Part print with two shaded views. Sizes in mm from the minimum x, y, z corner. A direction names the side the tool comes from. Round coordinates to 2 decimals unless told otherwise and drop trailing zeros. Write each loop counter-clockwise with the first axis right and the second up, starting at its lowest first coordinate (ties: lowest second). Pieces come first, ordered by that corner, then holes. Notation, with made-up numbers: (66.5, -31) -> (89.5, -31) arc R32 ccw to (89.5, -5) -> close; hole circle Ø11 at (6.5, 45.5). An arc over 180 degrees is marked (long way). Answer as CSV lines item,"result".
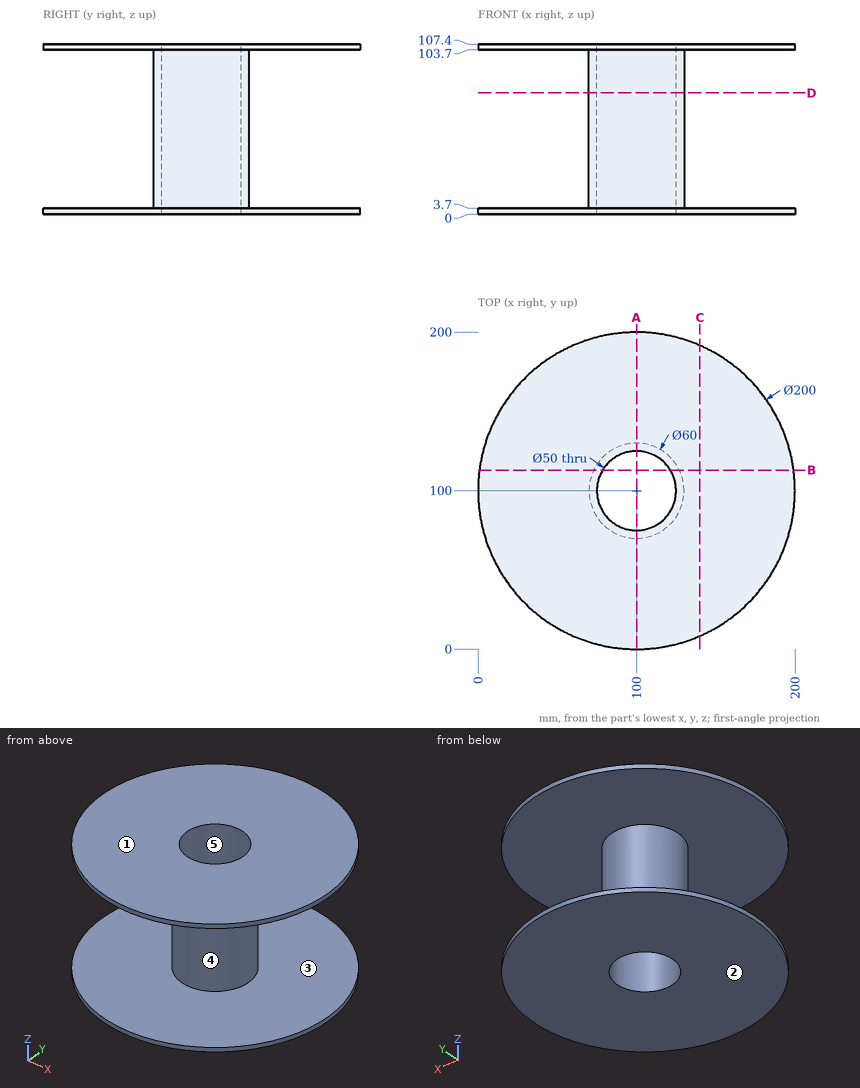
1. Mould opens along Z. For the marked faces 1, 2 and 3 say: +Z half, -Z half, draft (parallel to the pull), parting line (faces both ways), or undercut.
Results found:
face 1,"+Z half"
face 2,"-Z half"
face 3,"undercut"
2. Which spindle directions (+Z, -Z, +X, -X, +Y, -Y) get a long thin tool onto all of the face, cutting with end or side? Do the marked faces 4 and 5. Say none if no direction does.
Results found:
face 4,"none"
face 5,"+Z, -Z"
3. Cut at A-A, the plane x = 100. Write the cut outline in (y, z), then the cut area to 3 significant figures.
Results found:
outline,"(0, 0) -> (75, 0) -> (75, 107.4) -> (0, 107.4) -> (0, 103.7) -> (70, 103.7) -> (70, 3.7) -> (0, 3.7) -> close; (125, 0) -> (200, 0) -> (200, 3.7) -> (130, 3.7) -> (130, 103.7) -> (200, 103.7) -> (200, 107.4) -> (125, 107.4) -> close"
area,"2,110 mm2"
4. Probe line 1 along Y through (x, z) = (100, 31.5); line 2 along Z through (x, y) = (36.5, 45); line 3 along Y through (x, z) = (86, 93). List the from-to ranges inside material, lowest first.
Results found:
line 1,"y = 70 to 75, 125 to 130"
line 2,"z = 0 to 3.7, 103.7 to 107.4"
line 3,"y = 73.47 to 79.29, 120.71 to 126.53"
5. Cut at B-B, the plane y = 113. Write the cut outline in (x, z).
Results found:
outline,"(0.85, 0) -> (78.65, 0) -> (78.65, 107.4) -> (0.85, 107.4) -> (0.85, 103.7) -> (72.96, 103.7) -> (72.96, 3.7) -> (0.85, 3.7) -> close; (121.35, 0) -> (199.15, 0) -> (199.15, 3.7) -> (127.04, 3.7) -> (127.04, 103.7) -> (199.15, 103.7) -> (199.15, 107.4) -> (121.35, 107.4) -> close"
6. Drop flat-ended pins along their axis: pin 1 Ø5 at (y, z) = (102.5, 59) entering from +X; pin 2 Ø6 at (y, z) = (123, 95.5) entering from +X; pin 3 Ø12 at (y, z) = (96.5, 79) entering from -X; pin 4 Ø12 at (x, y) = (146, 129.5) entering from -Z. Give the stop position or say it passes through.
Results found:
pin 1,"stops at x = 130"
pin 2,"stops at x = 122.36"
pin 3,"stops at x = 70"
pin 4,"stops at z = 0"
7. Cut at C-C, the plane x = 140. Write the cut outline in (y, z).
Results found:
outline,"(8.35, 0) -> (191.65, 0) -> (191.65, 3.7) -> (8.35, 3.7) -> close; (8.35, 103.7) -> (191.65, 103.7) -> (191.65, 107.4) -> (8.35, 107.4) -> close"
8. Cut at D-D, the plane z = 76.5. Write the cut outline in (x, y).
Results found:
outline,"circle Ø60 at (100, 100); hole circle Ø50 at (100, 100)"
